For this review, use the dimensioned drawing (mm, ordinates from the lowest corner) and the shaded views. A direction names the side the tool comes from. Round coordinates to 2 decimals unless told otherwise and drop trailing zeros. Write each loop counter-clockwise with the first axis right and the second up, starting at its lowest first coordinate (ties: lowest second). Pieces come first, ordered by that corner, then holes. Notation, with made-up numbers: M 82,52.25 L 131,52.25 A26 cw 131,78.25 Z; hole C 5.5,-11 d11. An arc over 180 degrees is marked long. One line per question, with ' | ' between items.
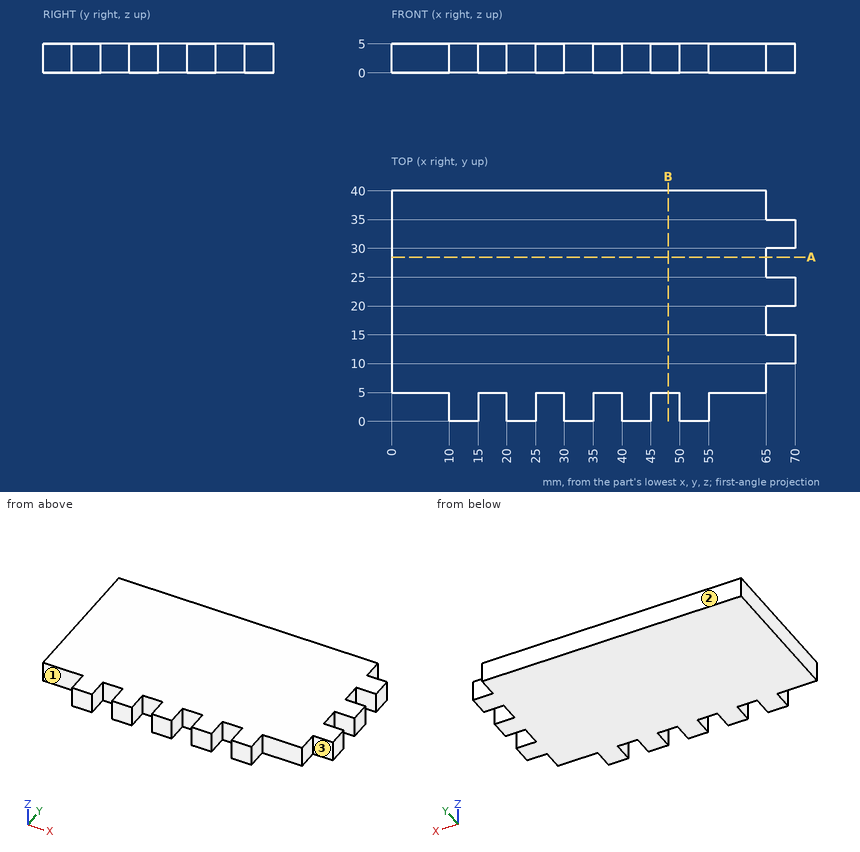
Item 1: Take a section at A-A (y = 28.5). Write out the cut boundary in (x, z), then the cut area to 3 significant figures.
Results:
outline: M 0,0 L 65,0 L 65,5 L 0,5 Z | area: 325 mm2
Item 2: To check wall thickness, follow line 1 along X through (y, z) = (2.5, 4.2); line 2 along Y through (x, z) = (29.5, 4.35); line 3 along X through (y, z) = (19, 1.95). State the ranges of each line that lie inside material, in increasing order. Write a range as from..to.
Results:
line 1: 10..15, 20..25, 30..35, 40..45, 50..55 | line 2: 5..40 | line 3: 0..65
Item 3: Take a section at B-B (x = 48). Write out the cut boundary in (y, z).
Results:
outline: M 5,0 L 40,0 L 40,5 L 5,5 Z
Item 4: Machinability: for the marked faces 1, 2 and 3, which of the approach directions +Z, -Z, +X, -X, +Y, -Y give a long, thin tool a straight path to every point of the face, cutting with its end or side? Answer none if there is none.
Results:
face 1: +Z, -Z, -X, -Y | face 2: +Z, -Z, +X, -X, +Y | face 3: +Z, -Z, +X, -Y
Item 5: Insertion check: pin 1 Ø2.5 at (x, z) = (27, 1.5) entering from -Y; pin 2 Ø2.5 at (y, z) = (3, 3) entering from +X; pin 3 Ø2.5 at (y, z) = (3.5, 2.5) entering from -X. Each pin has a flat end and moves straight along its axis. Give the tip position at first contact, or say it passes through.
Results:
pin 1: y = 5 | pin 2: x = 55 | pin 3: x = 10
